Work out the finished part from the listing and answer in its coordinate system (mm). A direction names the side the tool comes from. Coordinates: 2 decimals unless noted, no trailing zeros. Write each loop counter-clockwise with the first axis right and the second up, starting at its lowest first coordinate (ties: lowest second). Pieces come first, ordered by that corner, then holes. Notation, with made-up numbers: M 4,35 L 24,35 A12 ccw 24,54 Z; hole C 53.5,-29 d6. An arc over 180 degrees is marked long. Use CSV: the item, a comma, the result in double quotes.
Autodesk Inventor part; units mm, degrees
ref_plane "YZ Plane" through (0, 0, 0) normal (1, 0, 0) x (0, 1, 0)
ref_plane "XZ Plane" through (0, 0, 0) normal (0, 1, 0) x (-1, 0, 0)
ref_plane "XY Plane" through (0, 0, 0) normal (0, 0, 1) x (1, 0, 0)
sketch "Sketch1" plane through (0, 0, 0) normal (0, 0, 1) x (1, 0, 0)
  circle A0 centre (0, 0) radius 11
  circle A1 centre (0, 0) radius 4
  circle A2 centre (0, 0) radius 5.1201
  circle A3 centre (0, 0) radius 9.9838
  dimension "d0" = 22
  dimension "d1" = 8
extrude "Extrusion1" add sketch "Sketch1" along normal mid plane 7
extrude "Extrusion2" add sketch "Sketch1" along normal mid plane 6.5 contours A3
properties part number "8mmx22mm bearing"
Item 1: A tool of negligible diameter and unlimited length cuts with its end or side. For faces 4 (the face through (2, -10, 3.5)), 5 (the face through (-2, 5, -3.25)), 6 (the face through (-2, 5, 3.25)), from which of +Z, -Z, +X, -X, +Y, -Y can it reach the whole face along a straight path? Write none if from no direction.
Answer:
face 4,"+Z, +X, -X, +Y, -Y"
face 5,"-Z"
face 6,"+Z"
Item 2: The part is cut by section D-D (z = 0.5). Write down the section's boundary in (x, y), then the cut area to 3 significant figures.
Answer:
outline,"C 0,0 d22; hole C 0,0 d8"
area,"330 mm2"
Item 3: For a pull along X with two mould halves and no side action, classify faces 1 (the face through (-2.38, -10.74, 0.05)), 2 (the face through (-3, -3, 3.5)), 3 (the face through (-0.867, 3.905, -0.049)) as released by +X, released by -X, zero draft, split by the parting line, or undercut.
Answer:
face 1,"split by the parting line"
face 2,"zero draft"
face 3,"undercut"
Item 4: The part is cut by section C-C (x = 6). Write down the section's boundary in (y, z).
Answer:
outline,"M -9.22,-3.5 L -7.98,-3.5 L -7.98,-3.25 L 7.98,-3.25 L 7.98,-3.5 L 9.22,-3.5 L 9.22,3.5 L 7.98,3.5 L 7.98,3.25 L -7.98,3.25 L -7.98,3.5 L -9.22,3.5 Z"
Item 5: Given pin 1 (4 mm diameter, centred on x = 7, y = -1.5, fed in from +Z); pin 2 (1.5 mm diameter, centred on x = -1.5, z = -2, fed in from -Y); pin 3 (4 mm diameter, centred on y = 8, z = -1.5, fed in from -X), each flat-ended and moving along its own axis, determine where each tip first touches the part or whether it passes through.
Answer:
pin 1,"stops at z = 3.25"
pin 2,"stops at y = -10.97"
pin 3,"stops at x = -9.22"
Item 6: The part is cut by section A-A (y = 0). Write down the section's boundary in (x, z).
Answer:
outline,"M -11,-3.5 L -9.98,-3.5 L -9.98,-3.25 L -5.12,-3.25 L -5.12,-3.5 L -4,-3.5 L -4,3.5 L -5.12,3.5 L -5.12,3.25 L -9.98,3.25 L -9.98,3.5 L -11,3.5 Z; M 4,-3.5 L 5.12,-3.5 L 5.12,-3.25 L 9.98,-3.25 L 9.98,-3.5 L 11,-3.5 L 11,3.5 L 9.98,3.5 L 9.98,3.25 L 5.12,3.25 L 5.12,3.5 L 4,3.5 Z"
Item 7: Consider probe 1 along Y at (x, z) = (0, 3.35); probe 2 along Z at (x, y) = (-4.5, -4.5); probe 3 along Y at (x, z) = (0, -2). Determine where each line is inside the solid, lowest interval first.
Answer:
probe 1,"y = -11 to -9.98, -5.12 to -4, 4 to 5.12, 9.98 to 11"
probe 2,"z = -3.25 to 3.25"
probe 3,"y = -11 to -4, 4 to 11"
